```python
from build123d import *

# Parameters (mm, degrees)
EXTRUDE_1_DEPTH = 50


with BuildPart() as part:
    # 草图1 → 凸台-拉伸1 (new, symmetric)
    with BuildSketch(Plane.XY):
        with BuildLine():
            Line((12.49999999, 0), (-12.49999999, 0))
            ThreePointArc((-12.49999999, 0), (-14.267766942, -0.732233047), (-14.999999989, -2.499999998))
            Line((-14.999999989, -2.499999998), (-14.999999989, -172.500000002))
            ThreePointArc((-14.999999989, -172.500000002), (-14.267766942, -174.267766953), (-12.49999999, -175))
            Line((-12.49999999, -175), (-5.399999995, -175))
            ThreePointArc((-5.399999995, -175), (-5.187867961, -174.912132034), (-5.099999996, -174.7))
            Line((-5.099999996, -174.7), (-5.099999996, -174.300000001))
            ThreePointArc((-5.099999996, -174.300000001), (-5.01213203, -174.087867966), (-4.799999996, -174.000000001))
            Line((-4.799999996, -174.000000001), (-4.399999997, -174.000000001))
            ThreePointArc((-4.399999997, -174.000000001), (-4.187867962, -173.912132035), (-4.099999997, -173.700000001))
            Line((-4.099999997, -173.700000001), (-4.099999997, -173.100000001))
            ThreePointArc((-4.099999997, -173.100000001), (-4.187867962, -172.887867967), (-4.399999997, -172.800000002))
            Line((-4.399999997, -172.800000002), (-7.949999994, -172.800000002))
            ThreePointArc((-7.949999994, -172.800000002), (-8.162132028, -172.712132036), (-8.249999994, -172.500000002))
            Line((-8.249999994, -172.500000002), (-8.249999994, -169.929898991))
            ThreePointArc((-8.249999994, -169.929898991), (-8.227163853, -169.815093962), (-8.162132028, -169.717766957))
            Line((-8.162132028, -169.717766957), (-4.332233044, -165.887867973))
            ThreePointArc((-4.332233044, -165.887867973), (-4.234906039, -165.822836147), (-4.12010101, -165.800000007))
            Line((-4.12010101, -165.800000007), (4.12010101, -165.800000007))
            ThreePointArc((4.12010101, -165.800000007), (4.234906039, -165.822836147), (4.332233044, -165.887867973))
            Line((4.332233044, -165.887867973), (8.162132028, -169.717766957))
            ThreePointArc((8.162132028, -169.717766957), (8.227163854, -169.815093962), (8.249999994, -169.929898991))
            Line((8.249999994, -169.929898991), (8.249999994, -172.500000002))
            ThreePointArc((8.249999994, -172.500000002), (8.162132028, -172.712132036), (7.949999994, -172.800000002))
            Line((7.949999994, -172.800000002), (4.399999997, -172.800000002))
            ThreePointArc((4.399999997, -172.800000002), (4.187867963, -172.887867967), (4.099999997, -173.100000001))
            Line((4.099999997, -173.100000001), (4.099999997, -173.700000001))
            ThreePointArc((4.099999997, -173.700000001), (4.187867963, -173.912132035), (4.399999997, -174.000000001))
            Line((4.399999997, -174.000000001), (4.799999996, -174.000000001))
            ThreePointArc((4.799999996, -174.000000001), (5.01213203, -174.087867966), (5.099999996, -174.300000001))
            Line((5.099999996, -174.300000001), (5.099999996, -174.7))
            ThreePointArc((5.099999996, -174.7), (5.187867962, -174.912132034), (5.399999996, -175))
            Line((5.399999996, -175), (12.49999999, -175))
            ThreePointArc((12.49999999, -175), (14.267766942, -174.267766953), (14.999999989, -172.500000002))
            Line((14.999999989, -172.500000002), (14.999999989, -2.499999998))
            ThreePointArc((14.999999989, -2.499999998), (14.267766942, -0.732233047), (12.49999999, 0))
        make_face()
        with BuildLine():
            Line((10.999999989, -2), (-10.999999989, -2))
            ThreePointArc((-10.999999989, -2), (-12.414213551, -2.585786438), (-12.999999989, -4))
            Line((-12.999999989, -4), (-12.999999989, -52))
            ThreePointArc((-12.999999989, -52), (-12.414213551, -53.414213562), (-10.999999989, -54))
            Line((-10.999999989, -54), (10.999999989, -54))
            ThreePointArc((10.999999989, -54), (12.414213551, -53.414213562), (12.999999989, -52))
            Line((12.999999989, -52), (12.999999989, -4))
            ThreePointArc((12.999999989, -4), (12.414213551, -2.585786438), (10.999999989, -2))
        make_face(mode=Mode.SUBTRACT)
        with BuildLine():
            Line((10.999999989, -163.800000007), (-10.999999989, -163.800000007))
            ThreePointArc((-10.999999989, -163.800000007), (-12.414213551, -163.214213569), (-12.999999989, -161.800000007))
            Line((-12.999999989, -161.800000007), (-12.999999989, -112))
            ThreePointArc((-12.999999989, -112), (-12.414213551, -110.585786438), (-10.999999989, -110))
            Line((-10.999999989, -110), (10.999999989, -110))
            ThreePointArc((10.999999989, -110), (12.414213551, -110.585786438), (12.999999989, -112))
            Line((12.999999989, -112), (12.999999989, -161.800000007))
            ThreePointArc((12.999999989, -161.800000007), (12.414213551, -163.214213569), (10.999999989, -163.800000007))
        make_face(mode=Mode.SUBTRACT)
        with BuildLine():
            Line((-10.999999989, -56), (10.999999989, -56))
            ThreePointArc((10.999999989, -56), (12.414213551, -56.585786438), (12.999999989, -58))
            Line((12.999999989, -58), (12.999999989, -106))
            ThreePointArc((12.999999989, -106), (12.414213551, -107.414213562), (10.999999989, -108))
            Line((10.999999989, -108), (-10.999999989, -108))
            ThreePointArc((-10.999999989, -108), (-12.414213551, -107.414213562), (-12.999999989, -106))
            Line((-12.999999989, -106), (-12.999999989, -58))
            ThreePointArc((-12.999999989, -58), (-12.414213551, -56.585786438), (-10.999999989, -56))
        make_face(mode=Mode.SUBTRACT)
    extrude(amount=EXTRUDE_1_DEPTH, both=True)


solid = part.part
```
Part model, mm, in its own coordinate system. A direction names the side the tool comes from. Coordinates: 2 decimals unless noted, no trailing zeros. Write each loop counter-clockwise with the first axis right and the second up, starting at its lowest first coordinate (ties: lowest second). Pieces come first, ordered by that corner, then holes.
Item 1: Slice it at C-C (z = -39). Count the separate pieces of the cut face and the enclosed holes in it, and give its area (3 significant figures).
Item 2: Slice it at B-B (x = 0.25). Write the cut outline in (y, z), and give its area (3 significant figures).
Item 3: Pin check, flat tips, straight feed: pin 1 (0.5 mm diameter, centred on y = -173.5, z = -19, fed in from +X); pin 2 (0.5 mm diameter, centred on y = -173.5, z = 16, fed in from -X); pin 3 (4 mm diameter, centred on x = -0.5, z = 3.5, fed in from -Y); pin 4 (10 mm diameter, centred on x = 3.5, y = -48.5, fed in from -Z). Stop position of each tip, or through.
Item 4: Which spindle directions (+Z, -Z, +X, -X, +Y, -Y) get a long thin tool onto all of the face, cutting with end or side? Do faces 5 (the face through (-13, -28, 1)), 6 (the face through (0, 0, 1)). Say none if no direction does.
Item 5: Probe line 1 (Y direction, x = -2.25, z = -12); line 2 (Y direction, x = 11.25, z = -34.5); line 3 (X direction, y = -88.5, z = -24). List the from-to ranges inside material, lowest first.
Item 6: Slice it at A-A (y = -21.5). Write the cut outline in (x, z).
Item 7: Mould opens along Y. For faces 1 (the face through (0, -54, 1)), 2 (the face through (-9, -175, 1)), 3 (the face through (13.3, -100.1, 50)), 4 (the face through (13, -28, 1)) say: released by +Y, released by -Y, zero draft, split by the parting line, or undercut.
Results found:
1. separate pieces: 1
1. enclosed holes: 3
1. area: 1,030 mm2
2. outline: (-165.8, -50) - (-163.8, -50) - (-163.8, 50) - (-165.8, 50) - close; (-110, -50) - (-108, -50) - (-108, 50) - (-110, 50) - close; (-56, -50) - (-54, -50) - (-54, 50) - (-56, 50) - close; (-2, -50) - (0, -50) - (0, 50) - (-2, 50) - close
2. area: 800 mm2
3. pin 1: stops at x = 14.88
3. pin 2: stops at x = -14.88
3. pin 3: stops at y = -165.8
3. pin 4: passes through
4. face 5: +Z, -Z
4. face 6: +Z, -Z, +X, -X, +Y
5. line 1: y = -165.8 to -163.8, -110 to -108, -56 to -54, -2 to 0
5. line 2: y = -175 to -163.78, -110.02 to -107.98, -56.02 to -53.98, -2.02 to 0
5. line 3: x = -15 to -13, 13 to 15
6. outline: (-15, -50) - (-13, -50) - (-13, 50) - (-15, 50) - close; (13, -50) - (15, -50) - (15, 50) - (13, 50) - close
7. face 1: undercut
7. face 2: released by -Y
7. face 3: zero draft
7. face 4: undercut
